CAD build for the part. Positions are in the model's coordinates, mm. A direction names the side the tool comes from. Give positions to 0.01 mm unless a question says otherwise; leave off trailing zeros. Write each loop counter-clockwise with the first axis right and the second up, starting at its lowest first coordinate (ties: lowest second). Pieces come first, ordered by that corner, then holes. Notation, with made-up numbers: M 85.25,-40 L 122.25,-40 A12 cw 122.25,-20 Z; hole C 3.5,30 d4. An arc over 180 degrees is marked long. One line per question, with ' | ' between items. Start each with the question number.
1. Which spindle directions (+Z, -Z, +X, -X, +Y, -Y) get a long thin tool onto all of the face, cutting with end or side? Do faces 1 (the face through (1.972, 67.845, 10.867)), 2 (the face through (20, 107, 6)), 3 (the face through (22, 3, 4)), 4 (the face through (12.972, 73.458, 6.986)). Say none if no direction does.
2. Wall check: L1, parallel to X at y = 55, z = 7.75; L2, parallel to Y at x = 23.75, z = 14.5; L3, parallel to Y at x = 19.75, z = 1.5. Give the ranges that are in metal, low to high.
3. Cut at D-D, the plane x = 20. Write the cut outline in (y, z).
4. Cut at B-B, the plane z = 4. Write the cut outline in (x, y), then the cut area to 3 significant figures.
5. Pull direction X, two halves, no side cores. Call faces 5 (the face through (4, 36.5, 8.3)), 6 (the face through (20, 105, 10)), 7 (the face through (11, 70, 8)), 8 (the face through (11, 55, 13)): released by +X, released by -X, zero draft, split by the parting line, or undercut.
6. Flat gauge pins, fed straight in: pin 1 (1 mm diameter, centred on y = 66.5, z = 8.5, fed in from +X); pin 2 (5.5 mm diameter, centred on x = 20, z = 4, fed in from +Y); pin 3 (5 mm diameter, centred on x = 9, y = 22.5, fed in from +Z); pin 4 (3 mm diameter, centred on x = 17, y = 28.5, fed in from +Z). Where does each tip first touch, or does it go through?
7. Cut at C-C, the plane y = 88.5. Write the cut outline in (x, z), then the cut area to 3 significant figures.
8. Cut at A-A, the plane x = 7.5. Count the separate pieces of the cut face and the enclosed holes in it, then the cut area to 3 significant figures.
```python
from build123d import *

# Parameters (mm, degrees)
PAD001_DEPTH              = 4
BODY001_PLACEMENT_ANGLE   = 90
PAD_DEPTH                 = 4
BODY_PLACEMENT_ANGLE      = 90
CYLINDER011_R             = 2.25
CYLINDER011_DEPTH         = 15
CYLINDER010_R             = 4
CYLINDER010_DEPTH         = 4
CYLINDER009_R             = 2.25
CYLINDER009_DEPTH         = 15
CYLINDER008_R             = 4
CYLINDER008_DEPTH         = 4
CYLINDER007_R             = 1.7
CYLINDER007_DEPTH         = 15
CYLINDER006_R             = 3
CYLINDER006_DEPTH         = 3
FUSION003_PLACEMENT_ANGLE = 270
CYLINDER005_R             = 1.7
CYLINDER005_DEPTH         = 15
CYLINDER004_R             = 3
CYLINDER004_DEPTH         = 3
FUSION002_PLACEMENT_ANGLE = 90
CYLINDER001_R             = 5.25
CYLINDER001_DEPTH         = 7
CYLINDER_R                = 3.3
CYLINDER_DEPTH            = 20
ARRAY001_Y_COUNT          = 3
ARRAY001_Y_PITCH          = 33.5
BOX002_W                  = 10
BOX002_H                  = 100
BOX002_DEPTH              = 20
BOX001_W                  = 25
BOX001_H                  = 110
BOX001_DEPTH              = 20


with BuildPart() as body001:
    # Sketch001 → Pad001 (new body)
    with BuildSketch(Plane.XY):
        Polygon((4, 0), (2, 3.464102), (-2, 3.464102), (-4, 0), (-2, -3.464102), (2, -3.464102), align=None)
    extrude(amount=PAD001_DEPTH)


with BuildPart() as body001_1:
    # Body001 placement: moved
    add(body001.part.moved(Location((11, 71.75, 10))).rotate(Axis((11, 71.75, 10), (0, 1, 0)), BODY001_PLACEMENT_ANGLE))


with BuildPart() as fusion008:
    # Sketch → Pad (new body)
    with BuildSketch(Plane.XY):
        Polygon((4, 0), (2, 3.464102), (-2, 3.464102), (-4, 0), (-2, -3.464102), (2, -3.464102), align=None)
    extrude(amount=PAD_DEPTH)


with BuildPart() as fusion008_1:
    # Body placement: moved
    add(fusion008.part.moved(Location((11, 38.25, 10))).rotate(Axis((11, 38.25, 10), (0, 1, 0)), BODY_PLACEMENT_ANGLE))

    # Fusion008: union Body001
    add(body001_1.part)


with BuildPart() as cylinder011:
    # Cylinder011 → Cylinder011 (new body)
    with BuildSketch(Plane(origin=(0, 0, 0), x_dir=(0, 0, -1), z_dir=(1, 0, 0))):
        Circle(CYLINDER011_R)
    extrude(amount=CYLINDER011_DEPTH)


with BuildPart() as obj1:
    # Cylinder010 → Cylinder010 (new body)
    with BuildSketch(Plane(origin=(0, 0, 0), x_dir=(0, 0, -1), z_dir=(1, 0, 0))):
        Circle(CYLINDER010_R)
    extrude(amount=CYLINDER010_DEPTH)

    # Fusion006: union Cylinder011
    add(cylinder011.part)


with BuildPart() as obj1_1:
    # Fusion006 placement: moved
    add(obj1.part.moved(Location((0, 71.75, 10))))


with BuildPart() as cylinder009:
    # Cylinder009 → Cylinder009 (new body)
    with BuildSketch(Plane(origin=(0, 0, 0), x_dir=(0, 0, -1), z_dir=(1, 0, 0))):
        Circle(CYLINDER009_R)
    extrude(amount=CYLINDER009_DEPTH)


with BuildPart() as fusion007:
    # Cylinder008 → Cylinder008 (new body)
    with BuildSketch(Plane(origin=(0, 0, 0), x_dir=(0, 0, -1), z_dir=(1, 0, 0))):
        Circle(CYLINDER008_R)
    extrude(amount=CYLINDER008_DEPTH)

    # Fusion005: union Cylinder009
    add(cylinder009.part)


with BuildPart() as fusion007_1:
    # Fusion005 placement: moved
    add(fusion007.part.moved(Location((0, 38.25, 10))))

    # Fusion007: union obj1
    add(obj1_1.part)


with BuildPart() as cylinder007:
    # Cylinder007 → Cylinder007 (new body)
    with BuildSketch(Plane.XY):
        Circle(CYLINDER007_R)
    extrude(amount=CYLINDER007_DEPTH)


with BuildPart() as obj2:
    # Cylinder006 → Cylinder006 (new body)
    with BuildSketch(Plane.XY.offset(12)):
        Circle(CYLINDER006_R)
    extrude(amount=CYLINDER006_DEPTH)

    # Fusion003: union Cylinder007
    add(cylinder007.part)


with BuildPart() as obj2_1:
    # Fusion003 placement: moved
    add(obj2.part.moved(Location((20, 95, 4))).rotate(Axis((20, 95, 4), (1, 0, 0)), FUSION003_PLACEMENT_ANGLE))


with BuildPart() as cylinder005:
    # Cylinder005 → Cylinder005 (new body)
    with BuildSketch(Plane.XY):
        Circle(CYLINDER005_R)
    extrude(amount=CYLINDER005_DEPTH)


with BuildPart() as fusion004:
    # Cylinder004 → Cylinder004 (new body)
    with BuildSketch(Plane.XY.offset(12)):
        Circle(CYLINDER004_R)
    extrude(amount=CYLINDER004_DEPTH)

    # Fusion002: union Cylinder005
    add(cylinder005.part)


with BuildPart() as fusion004_1:
    # Fusion002 placement: moved
    add(fusion004.part.moved(Location((20, 15, 4))).rotate(Axis((20, 15, 4), (1, 0, 0)), FUSION002_PLACEMENT_ANGLE))

    # Fusion004: union obj2
    add(obj2_1.part)


with BuildPart() as cylinder001:
    # Cylinder001 → Cylinder001 (new body)
    with BuildSketch(Plane.XY.offset(13)):
        Circle(CYLINDER001_R)
    extrude(amount=CYLINDER001_DEPTH)


with BuildPart() as array001:
    # Cylinder → Cylinder (new body)
    with BuildSketch(Plane.XY):
        Circle(CYLINDER_R)
    extrude(amount=CYLINDER_DEPTH)

    # Fusion: union Cylinder001
    add(cylinder001.part)


with BuildPart() as array001_1:
    # Fusion placement: moved
    add(array001.part.moved(Location((7.5, 0, 0))))

    # Array001 Y: Array001 ×3


with BuildPart() as array001_2:
    add(array001_1.part)
    with Locations(*[(0, i * ARRAY001_Y_PITCH, 0) for i in range(1, ARRAY001_Y_COUNT)]):
        add(array001_1.part)


with BuildPart() as array001_3:
    # Array001 placement: moved
    add(array001_2.part.moved(Location((0, 21.5, 0))))


with BuildPart() as cube002:
    # Box002 → Box002 (new body)
    with BuildSketch(Plane(origin=(15, 5, 0), x_dir=(1, 0, 0), z_dir=(0, 0, 1))):
        with Locations((5, 50)):
            Rectangle(BOX002_W, BOX002_H)
    extrude(amount=BOX002_DEPTH)


with BuildPart() as variablechuck:
    # Box001 → Box001 (new body)
    with BuildSketch(Plane.XY):
        with Locations((12.5, 55)):
            Rectangle(BOX001_W, BOX001_H)
    extrude(amount=BOX001_DEPTH)

    # Cut: cut Cube002
    add(cube002.part, mode=Mode.SUBTRACT)

    # Cut001: cut Array001
    add(array001_3.part, mode=Mode.SUBTRACT)

    # Cut004: cut Fusion004
    add(fusion004_1.part, mode=Mode.SUBTRACT)

    # Cut005: cut Fusion007
    add(fusion007_1.part, mode=Mode.SUBTRACT)

    # Cut006: cut Fusion008
    add(fusion008_1.part, mode=Mode.SUBTRACT)


solid = variablechuck.part
```
Here are the results:
1) face 1: -X | face 2: +Y | face 3: -Y | face 4: +X
2) L1: 0 to 4.2, 10.8 to 15 | L2: 0 to 5, 105 to 110 | L3: 3 to 5, 105 to 107
3) outline: M 0,0 L 5,0 L 5,2.3 L 3,2.3 L 3,1 L 0,1 Z; M 0,7 L 3,7 L 3,5.7 L 5,5.7 L 5,20 L 0,20 Z; M 105,0 L 110,0 L 110,1 L 107,1 L 107,2.3 L 105,2.3 Z; M 105,5.7 L 107,5.7 L 107,7 L 110,7 L 110,20 L 105,20 Z
4) outline: M 0,0 L 17,0 L 17,3 L 18.3,3 L 18.3,5 L 15,5 L 15,105 L 18.3,105 L 18.3,107 L 17,107 L 17,110 L 0,110 Z; M 21.7,3 L 23,3 L 23,0 L 25,0 L 25,5 L 21.7,5 Z; M 21.7,105 L 25,105 L 25,110 L 23,110 L 23,107 L 21.7,107 Z; hole C 7.5,21.5 d6.6; hole C 7.5,55 d6.6; hole C 7.5,88.5 d6.6 | area: 1,600 mm^2
5) face 5: released by -X | face 6: zero draft | face 7: released by +X | face 8: undercut
6) pin 1: x = 15 | pin 2: y = 107 | pin 3: z = 13 | pin 4: through
7) outline: M 0,0 L 4.2,0 L 4.2,13 L 2.25,13 L 2.25,20 L 0,20 Z; M 10.8,0 L 15,0 L 15,20 L 12.75,20 L 12.75,13 L 10.8,13 Z | area: 141 mm^2
8) separate pieces: 4 | enclosed holes: 2 | area: 1,690 mm^2
